from build123d import *

# Parameters (mm, degrees)
F0_W     = 160
F0_H     = 40
F1_DEPTH = 32
F3_DEPTH = 40.001
F4_W     = 6
F4_H     = 34
F4_W_2   = 14
F5_DEPTH = 25


with BuildPart() as f1:
    # F0 (on Top) → F1 (new body)
    with BuildSketch(Plane.XY):
        Rectangle(F0_W, F0_H)
    extrude(amount=F1_DEPTH)

    # F2 (on face) → F3 (cut, through all)
    with BuildSketch(Plane.XZ.offset(20)):
        with BuildLine():
            ThreePointArc((-80, 26), (-78.2426406871, 30.2426406871), (-74, 32))
            Line((-74, 32), (-80, 32))
            Line((-80, 32), (-80, 26))
        make_face()
        with BuildLine():
            Line((80, 32), (74, 32))
            ThreePointArc((74, 32), (78.2426406871, 30.2426406871), (80, 26))
            Line((80, 26), (80, 32))
        make_face()
    extrude(amount=-F3_DEPTH, mode=Mode.SUBTRACT)

    # F4 (on face) → F5 (cut)
    with BuildSketch(Plane.XY.offset(32)):
        with Locations((77, 0)):
            Rectangle(F4_W, F4_H)
        with Locations((-67, 0)):
            Rectangle(F4_W_2, F4_H)
        with Locations((67, 0)):
            Rectangle(F4_W_2, F4_H)
        with Locations((-77, 0)):
            Rectangle(F4_W, F4_H)
    extrude(amount=-F5_DEPTH, mode=Mode.SUBTRACT)


solid = f1.part
Model file for the job. Use its own axes, mm. A direction names the side the tool comes from. Round coordinates to 2 decimals unless told otherwise and drop trailing zeros. Loops run counter-clockwise (first coordinate to the right, second up) from the corner with the lowest first, then second, coordinate; pieces in that order, holes last. Notation, with made-up numbers: (-32, 76) -> (12, 76) arc R16 ccw to (12, 86) -> close; hole circle Ø10 at (75, 55.25). An arc over 180 degrees is marked (long way). Answer as CSV lines item,"result". Start each with the question number.
1) Probe line 1 along Y through (x, z) = (66, 30.5); line 2 along X through (y, z) = (6, 18.5); line 3 along Z through (x, y) = (62, 6.5). List the from-to ranges inside material, lowest first.
2) Tool access for faces 1 (the face through (-70, -17, 20)), 2 (the face through (80, 0, 4)), 3 (the face through (70, 0, 7)): list every direction of +Z, -Z, +X, -X, +Y, -Y with a clear straight run to the whole face (end or side of a thin tool).
3) Slice it at B-B (y = 13.5). List the corners of the cut face in (x, z).
4) Slice it at A-A (z = 22.5). List the corners of the cut face in (x, y).
5) Pin check, flat tips, straight feed: P1, Ø6, axis at x = -73.5, y = -6, coming from the +Z side; P2, Ø4, axis at y = 0.5, z = 25, coming from the +X side; P3, Ø7.5, axis at y = -5.5, z = 20.5, coming from the -X side. Stop position of each tip, or through.
6) Mould opens along Y. For faces 4 (the face through (-1, 20, 16)), 5 (the face through (-60, 0, 20)), 6 (the face through (-70, 17, 20)), 7 (the face through (-78.289, -18.521, 30.196)) say: +Y half, -Y half, draft (parallel to the pull), parting line (faces both ways), or undercut.
Filled in:
1,line 1,"y = -20 to -17, 17 to 20"
1,line 2,"x = -60 to 60"
1,line 3,"z = 0 to 7"
2,face 1,"+Z, -X"
2,face 2,"+Z, -Z, +X, +Y, -Y"
2,face 3,"+Z, +X"
3,outline,"(-80, 0) -> (80, 0) -> (80, 7) -> (60, 7) -> (60, 32) -> (-60, 32) -> (-60, 7) -> (-80, 7) -> close"
4,outline,"(-80, -20) -> (80, -20) -> (80, -17) -> (60, -17) -> (60, 17) -> (80, 17) -> (80, 20) -> (-80, 20) -> (-80, 17) -> (-60, 17) -> (-60, -17) -> (-80, -17) -> close"
5,P1,"stops at z = 7"
5,P2,"stops at x = 60"
5,P3,"stops at x = -60"
6,face 4,"+Y half"
6,face 5,"undercut"
6,face 6,"undercut"
6,face 7,"draft"
